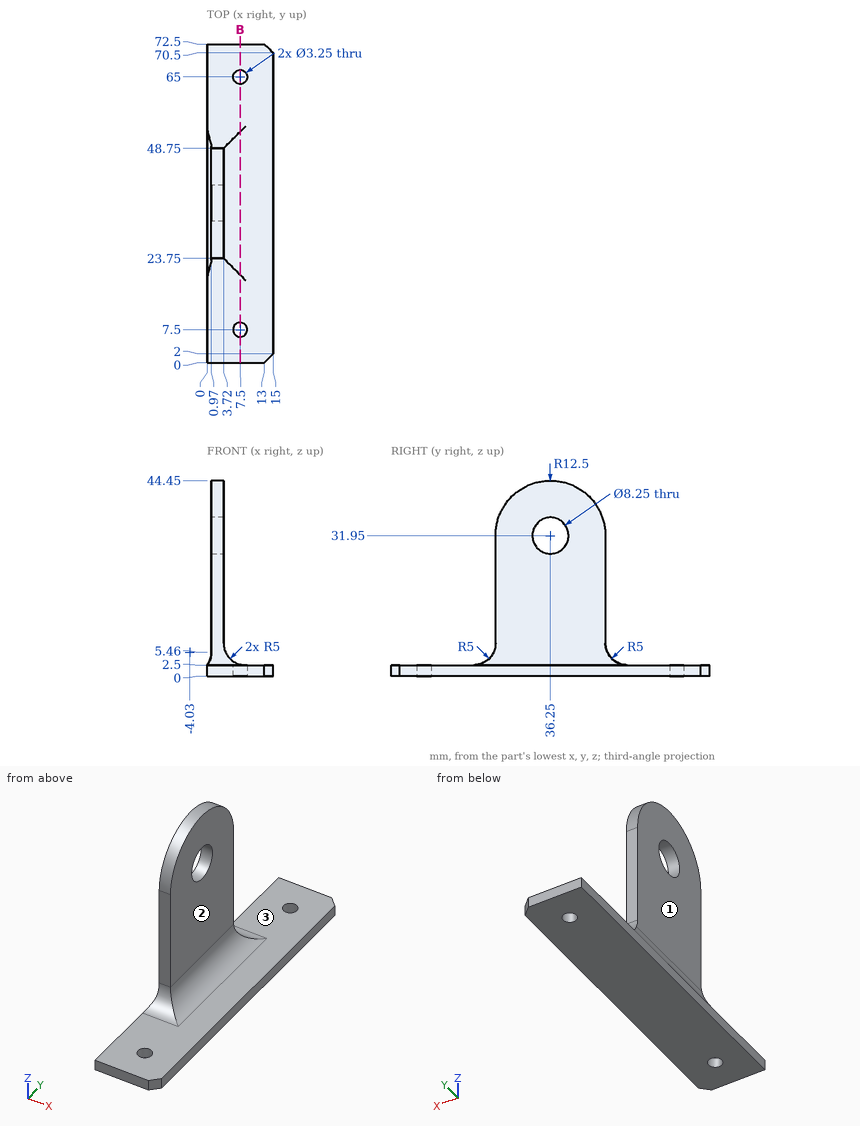
Can you work these out from the drawing? Everything is in mm from the part's minimum corner. A direction names the side the tool comes from. Round coordinates to 2 decimals unless told otherwise and drop trailing zeros. Write item = value, one per line.
1. I need wall thicknesses on probe 1 along Y at (x, z) = (7.5, 0.9) (1 decimal); probe 2 along X at (y, z) = (7.5, 1.25) (1 decimal); probe 3 along X at (y, z) = (47, 19). Which ranges of each line are inside material? Lowest first, please.
Results below:
probe_1 = 0 to 5.9, 9.1 to 63.4, 66.6 to 72.5
probe_2 = 0 to 5.9, 9.1 to 15
probe_3 = 0.97 to 3.72
2. Will these pins go through, and if not, where does the flat tip stop? P1, Ø12.5, axis at y = 35.5, z = 27, coming from the +X side; P2, Ø0.8, axis at x = 2, z = 16, coming from the -Y side; P3, Ø20.5, axis at y = 41.5, z = 22, coming from the -X side.
Results below:
P1 = 3.72
P2 = 23.75
P3 = 0.97
3. I want a section at B-B, the plane x = 7.5. Count the separate pieces of the cut face and the enclosed holes in it, and give its area (3 significant figures).
Results below:
separate_pieces = 3
enclosed_holes = 0
area = 170 mm²
4. Which directions (+Z, -Z, +X, -X, +Y, -Y) give clear straight access to the entire face, cutting with the end or side of a thin tool? Please do the marked faces 1, 2 and 3.
Results below:
face_1 = +Z, -X, +Y, -Y
face_2 = +Z, +X, +Y, -Y
face_3 = +Z, +X
